```python
from build123d import *

# Parameters (mm, degrees)
F0_W     = 300
F0_H     = 300
F0_W_2   = 140
F0_H_2   = 35
F1_DEPTH = 5
F2_R     = 1.25
F3_DEPTH = 5.001


with BuildPart() as f1:
    # F0 (on Top) → F1 (new body)
    with BuildSketch(Plane.XY):
        Rectangle(F0_W, F0_H)
        with Locations((0, 52.5)):
            Rectangle(F0_W_2, F0_H_2, mode=Mode.SUBTRACT)
    extrude(amount=F1_DEPTH)

    # F2 (on face) → F3 (cut, through all)
    with BuildSketch(Plane.XY.offset(5)):
        with Locations((-135, 135)):
            Circle(F2_R)
        with Locations((135, 135)):
            Circle(F2_R)
        with Locations((-135, -135)):
            Circle(F2_R)
        with Locations((135, -135)):
            Circle(F2_R)
        with Locations((-105, -135)):
            Circle(F2_R)
        with Locations((105, -135)):
            Circle(F2_R)
        with Locations((105, 135)):
            Circle(F2_R)
        with Locations((-105, 135)):
            Circle(F2_R)
    extrude(amount=-F3_DEPTH, mode=Mode.SUBTRACT)


solid = f1.part
```
Check sheet for the modelled part. Datum: model origin and axes. Units: mm. Coordinates: 2 decimals unless noted, no trailing zeros. Order: outer loops, then holes, each group sorted by start corner. A loop starts at its lowest first (then second) coordinate and runs counter-clockwise, first axis right, second up. Notation, with made-up numbers: M -21.5,67 L 4.5,67 A29 ccw 4.5,89 Z; hole C 39.5,42.5 d4. An arc over 180 degrees is marked long. One line per question, with ' | ' between items. Start each with the question number.
Item 1: Material ranges on line 1 (Y direction, x = 105, z = 3.1); line 2 (X direction, y = 135, z = 2.4); line 3 (Y direction, x = -69, z = 1.45), recorded low to high.
Item 2: Sectioned sample at A-A on x = 40.5. Record the cut outline in (y, z).
Item 3: Sectioned sample at B-B on z = 2.25. Count the separate pieces of the cut face and the enclosed holes in it, and give its area (3 significant figures).
Answer below:
1) line 1: y = -150 to -136.25, -133.75 to 133.75, 136.25 to 150 | line 2: x = -150 to -136.25, -133.75 to -106.25, -103.75 to 103.75, 106.25 to 133.75, 136.25 to 150 | line 3: y = -150 to 35, 70 to 150
2) outline: M -150,0 L 35,0 L 35,5 L -150,5 Z; M 70,0 L 150,0 L 150,5 L 70,5 Z
3) separate pieces: 1 | enclosed holes: 9 | area: 85,100 mm^2
